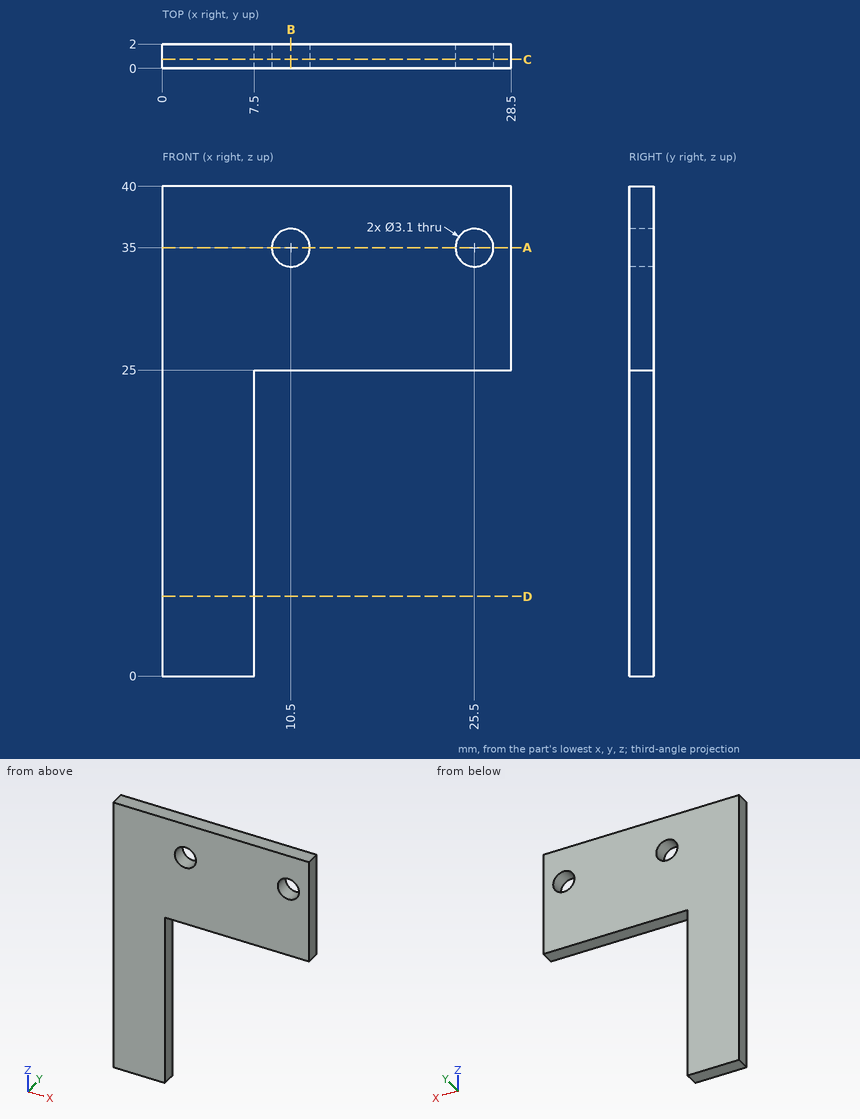
Geometry: see drawing. Coordinates: mm, zero at the bounding-box minimum. Give positions to 0.01 mm unless a question says otherwise; leave off trailing zeros. Order: outer loops, then holes, each group sorted by start corner. A loop starts at its lowest first (then second) coordinate and runs counter-clockwise, first axis right, second up.
Q1. Section C-C on y = 0.75. Output: boundary loops of the cut face in (x, z).
Checked values:
outline: (0, 0) - (7.5, 0) - (7.5, 25) - (28.5, 25) - (28.5, 40) - (0, 40) - close; hole circle Ø3.1 at (10.5, 35); hole circle Ø3.1 at (25.5, 35)
Q2. Section B-B on x = 10.5. Output: boundary loops of the cut face in (y, z), and give its area (3 significant figures).
Checked values:
outline: (0, 25) - (2, 25) - (2, 33.45) - (0, 33.45) - close; (0, 36.55) - (2, 36.55) - (2, 40) - (0, 40) - close
area: 23.8 mm2
Q3. Section D-D on z = 6.5. Output: boundary loops of the cut face in (x, y).
Checked values:
outline: (0, 0) - (7.5, 0) - (7.5, 2) - (0, 2) - close
Q4. Section A-A on z = 35. Output: boundary loops of the cut face in (x, y), and give its area (3 significant figures).
Checked values:
outline: (0, 0) - (8.95, 0) - (8.95, 2) - (0, 2) - close; (12.05, 0) - (23.95, 0) - (23.95, 2) - (12.05, 2) - close; (27.05, 0) - (28.5, 0) - (28.5, 2) - (27.05, 2) - close
area: 44.6 mm2
Q5. Ray query, probe 1 along X at (y, z) = (0.55, 35); probe 2 along Z at (x, y) = (10.5, 1.1); probe 3 along X at (y, z) = (0.7, 24.5). Return the intervals inside material, ascending.
Checked values:
probe 1: x = 0 to 8.95, 12.05 to 23.95, 27.05 to 28.5
probe 2: z = 25 to 33.45, 36.55 to 40
probe 3: x = 0 to 7.5
